Can you work these out from the model? Positions are in its coordinate system, mm. Face numbers are marked on the shaded views. A direction names the side the tool comes from. Give positions to 0.01 mm unless a question says otherwise; leave off trailing zeros. Write each loop counter-clockwise with the first axis right and the second up, starting at its lowest first coordinate (ties: lowest second). Pieces come first, ordered by that corner, then holes. Notation, with made-up numbers: M 18,10 L 67,10 A33 ccw 67,41 Z; hole C 44.25,35 d3. An arc over 180 degrees is marked long. Write each question's results on one line, items separated by ' | '.
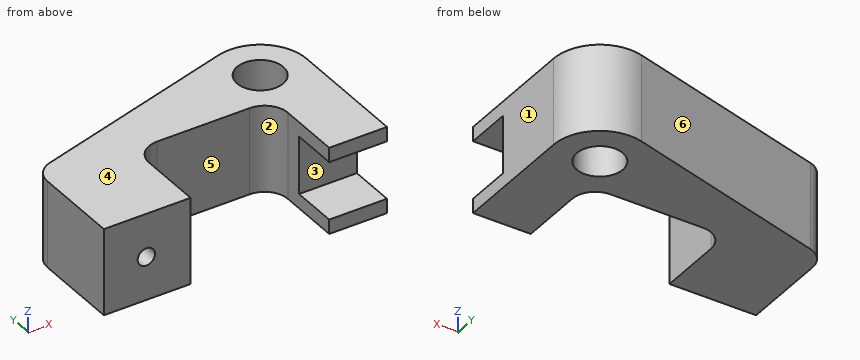
from build123d import *

# Parameters (mm, degrees)
EXTRUDE_1_DEPTH          = 15
FILLET_1_R               = 8
FILLET_2_R               = 4
SKETCH_2_R               = 4
CUT_EXTRUDE_1_DEPTH      = 46.20636026
FILLET_3_R               = 4
FILLET_4_R               = 4
SKETCH_3_R               = 1.5
CUT_EXTRUDE_2_DEPTH      = 10
CUT_EXTRUDE_3_DEPTH      = 61.351439793
CUT_EXTRUDE_3_DEPTH_BACK = 20
SKETCH_4_W               = 10
SKETCH_4_H               = 8


with BuildPart() as part:
    # 草图1 → 凸台-拉伸1 (new body)
    with BuildSketch(Plane.XY):
        Polygon((-20.674768795, 2.485242081), (-5.674768795, 2.485242081), (-5.674768795, 17.485242081), (18.325231205, 17.485242081), (18.325231205, 2.485242081), (28.325231205, 2.485242081), (28.325231205, 34.485242081), (-20.674768795, 20.485242081), align=None)
    extrude(amount=EXTRUDE_1_DEPTH)

    # 圆角1
    fillet_1_edges = [part.edges().sort_by_distance(p)[0] for p in [
        (28.325231205, 34.485242081, 7.5),
    ]]
    fillet(fillet_1_edges, radius=FILLET_1_R)

    # 圆角2
    fillet_2_edges = [part.edges().sort_by_distance(p)[0] for p in [
        (-20.674768795, 20.485242081, 7.5),
    ]]
    fillet(fillet_2_edges, radius=FILLET_2_R)

    # 草图2 → 切除-拉伸1 (cut, through all)
    with BuildSketch(Plane.XY.offset(15)):
        with Locations((20.325231205, 23.879402207)):
            Circle(SKETCH_2_R)
    extrude(amount=-CUT_EXTRUDE_1_DEPTH, mode=Mode.SUBTRACT)

    # 圆角3
    fillet_3_edges = [part.edges().sort_by_distance(p)[0] for p in [
        (-5.674768795, 17.485242081, 7.5),
    ]]
    fillet(fillet_3_edges, radius=FILLET_3_R)

    # 圆角4
    fillet_4_edges = [part.edges().sort_by_distance(p)[0] for p in [
        (18.325231205, 17.485242081, 7.5),
    ]]
    fillet(fillet_4_edges, radius=FILLET_4_R)

    # 草图3 → 切除-拉伸2 (cut)
    with BuildSketch(Plane.XZ.offset(-2.485242081)):
        with Locations(Location((-13.323141104, 7.5, 0), (0, 0, 270))):
            Circle(SKETCH_3_R)
    extrude(amount=-CUT_EXTRUDE_2_DEPTH, mode=Mode.SUBTRACT)

    # 草图4 → 切除-拉伸3 (cut, two sides: drawn at the far end of the back side and taken through both)
    with BuildSketch(Plane(origin=(28.325231205, 0, 0), x_dir=(0, 0, -1), z_dir=(1, 0, 0)).offset(-CUT_EXTRUDE_3_DEPTH_BACK)):
        with Locations((-7.5, 6.485242081)):
            Rectangle(SKETCH_4_W, SKETCH_4_H)
    extrude(amount=CUT_EXTRUDE_3_DEPTH + CUT_EXTRUDE_3_DEPTH_BACK, mode=Mode.SUBTRACT)


solid = part.part
Item 1: I'm going to push flat-ended pins straight in: pin 1 (9 mm diameter, centred on y = 6, z = 9, fed in from +X); pin 2 (0.9 mm diameter, centred on x = -14, z = 7.5, fed in from -Y); pin 3 (2.5 mm diameter, centred on x = -13.32, z = 7.5, fed in from +Y); pin 4 (8 mm diameter, centred on y = 22, z = 11.5, fed in from -X). Where does each tip first touch, or does it pass through?
Geometry says:
pin 1: stops at x = 28.33 | pin 2: stops at y = 12.49 | pin 3: stops at y = 22.94 | pin 4: stops at x = -20.64
Item 2: I want a section at D-D, the plane z = 14. Please give me the cut outline in (x, y), and give its area (3 significant figures).
Geometry says:
outline: M -20.67,2.49 L -5.67,2.49 L -5.67,13.49 A4 cw -1.67,17.49 L 14.33,17.49 A4 cw 18.33,13.49 L 18.33,2.49 L 28.33,2.49 L 28.33,23.88 A8 ccw 18.13,31.57 L -17.77,21.31 A4 ccw -20.67,17.47 Z; hole C 20.33,23.88 d8 | area: 794 mm2
Item 3: I want a section at B-B, the plane y = 25.75. Please give me the cut outline in (x, z).
Geometry says:
outline: M -2.25,0 L 16.79,0 L 16.79,15 L -2.25,15 Z; M 23.86,0 L 28.1,0 L 28.1,15 L 23.86,15 Z
Item 4: For the marked faces 1, 2 and 3, which set-ups out of +Z, -Z, +X, -X, +Y, -Y let a thin tool reach every point of the face, with its end or its side?
Geometry says:
face 1: +Z, -Z, +X, +Y, -Y | face 2: +Z, -Z, -Y | face 3: +X, -Y
Item 5: Thinking about a two-plate mould opening in X: for the marked faces 4, 5 and 6, which applies, +X half, -X half, draft (parallel to the pull), parting line (faces both ways), or undercut?
Geometry says:
face 4: draft | face 5: undercut | face 6: -X half
Item 6: I want a section at C-C, the plane y = 9.25. Please give me the cut outline in (x, z), and give its area (3 significant figures).
Geometry says:
outline: M -20.67,0 L -5.67,0 L -5.67,15 L -20.67,15 Z; M 18.33,0 L 28.33,0 L 28.33,2.5 L 18.33,2.5 Z; M 18.33,12.5 L 28.33,12.5 L 28.33,15 L 18.33,15 Z; hole C -13.32,7.5 d3 | area: 268 mm2
Item 7: If I drill on line 1 (X direction, y = 5.25, z = 7.5); line 2 (X direction, y = 7.75, z = 3.5); line 3 (X direction, y = 12.5, z = 14.25), over which ranges is the centre line in solid material (lowest first)? Write a range as from..to.
Geometry says:
line 1: x = -20.67..-14.82, -11.82..-5.67 | line 2: x = -20.67..-5.67 | line 3: x = -20.67..-5.67, 18.33..28.33
Item 8: I want a section at A-A, the plane z = 7.5. Please give me the cut outline in (x, y), and give its area (3 significant figures).
Geometry says:
outline: M -20.67,2.49 L -14.82,2.49 L -14.82,12.49 L -11.82,12.49 L -11.82,2.49 L -5.67,2.49 L -5.67,13.49 A4 cw -1.67,17.49 L 14.33,17.49 A4 cw 18.33,13.49 L 18.33,10.49 L 28.33,10.49 L 28.33,23.88 A8 ccw 18.13,31.57 L -17.77,21.31 A4 ccw -20.67,17.47 Z; hole C 20.33,23.88 d8 | area: 684 mm2
